Work out the finished part from the listing and answer in its coordinate system (mm). Face numbers are marked on the shaded views. A direction names the side the tool comes from. Give positions to 0.01 mm unless a question says otherwise; leave off trailing zeros. Loops run counter-clockwise (first coordinate to the right, second up) from the corner with the lowest first, then second, coordinate; pieces in that order, holes last. Notation, with made-up numbers: M 87.25,-18.5 L 101.25,-18.5 A18 ccw 101.25,-3.5 Z; hole C 0,61.5 d6. An arc over 180 degrees is marked long. Use a Markdown table: item, result.
```python
from build123d import *

# Parameters (mm, degrees)
SKETCH1_W               = 31.2625
SKETCH1_H               = 55
BOSS_EXTRUDE1_DEPTH     = 3.175
SKETCH2_R               = 1.5
CUT_EXTRUDE1_DEPTH      = 10
LPATTERN1_COUNT         = 3
LPATTERN1_PITCH         = 10
LPATTERN1_COL_COUNT     = 3
LPATTERN1_COL_PITCH     = 10
SKETCH3_W               = 6.35
SKETCH3_H               = 3.175
CUT_EXTRUDE2_DEPTH      = 10
LPATTERN2_COUNT         = 5
LPATTERN2_PITCH         = 6.35
LPATTERN2_COL_COUNT     = 5
LPATTERN2_COL_PITCH     = 6.35
SKETCH4_W               = 3.175
SKETCH4_H               = 3.6875
SKETCH4_H_2             = 3.175
CUT_EXTRUDE3_DEPTH      = 10
SKETCH5_W               = 6.35
SKETCH5_H               = 55
CUT_EXTRUDE4_DEPTH      = 10
SKETCH6_W               = 3.175
SKETCH6_H               = 3.175
CUT_EXTRUDE5_DEPTH      = 10
LPATTERN3_COUNT         = 2
LPATTERN3_PITCH         = 6.35
LPATTERN3_COUNT_DIR2    = 2
LPATTERN3_PITCH_DIR2    = 6.35
SKETCH7_W               = 5.8625
SKETCH7_H               = 3.175
CUT_EXTRUDE6_DEPTH      = 10
MIRROR1_COPY_1_SKETCH_W = 3.175
MIRROR1_COPY_1_SKETCH_H = 3.175
MIRROR1_COPY_1_DEPTH    = 10
MIRROR1_COPY_2_SKETCH_W = 3.175
MIRROR1_COPY_2_SKETCH_H = 3.175
MIRROR1_COPY_2_DEPTH    = 10
MIRROR1_COPY_3_SKETCH_W = 3.175
MIRROR1_COPY_3_SKETCH_H = 3.175
MIRROR1_COPY_3_DEPTH    = 10
SKETCH8_W               = 21.7375
SKETCH8_H               = 3.175
SKETCH8_W_2             = 3.175
SKETCH8_H_2             = 41.275
SKETCH8_W_3             = 15.875
CUT_EXTRUDE7_DEPTH      = 10
CUT_EXTRUDE8_DEPTH      = 10
LPATTERN4_COUNT         = 5
LPATTERN4_PITCH         = 10


with BuildPart() as part:
    # Sketch1 → Boss-Extrude1 (new body)
    with BuildSketch(Plane.XY):
        Rectangle(SKETCH1_W, SKETCH1_H)
    extrude(amount=BOSS_EXTRUDE1_DEPTH)

    # Sketch2 → Cut-Extrude1 (cut)
    with BuildSketch(Plane.XY.offset(3.175)):
        Circle(SKETCH2_R)
    cut_extrude1 = extrude(amount=-CUT_EXTRUDE1_DEPTH, mode=Mode.SUBTRACT)

    # LPattern1: Cut-Extrude1 ×3
    with Locations(*[(0, i * LPATTERN1_PITCH, 0) for i in range(1, LPATTERN1_COUNT)]):
        add(cut_extrude1, mode=Mode.SUBTRACT)

    # LPattern1 col: Cut-Extrude1 ×3
    with Locations(*[(0, -i * LPATTERN1_COL_PITCH, 0) for i in range(1, LPATTERN1_COL_COUNT)]):
        add(cut_extrude1, mode=Mode.SUBTRACT)

    # Sketch3 → Cut-Extrude2 (cut)
    with BuildSketch(Plane.XY.offset(3.175)):
        with Locations((15.63125, -3.175)):
            Rectangle(SKETCH3_W, SKETCH3_H)
    cut_extrude2 = extrude(amount=-CUT_EXTRUDE2_DEPTH, mode=Mode.SUBTRACT)

    # LPattern2: Cut-Extrude2 ×5
    with Locations(*[(0, i * LPATTERN2_PITCH, 0) for i in range(1, LPATTERN2_COUNT)]):
        add(cut_extrude2, mode=Mode.SUBTRACT)

    # LPattern2 col: Cut-Extrude2 ×5
    with Locations(*[(0, -i * LPATTERN2_COL_PITCH, 0) for i in range(1, LPATTERN2_COL_COUNT)]):
        add(cut_extrude2, mode=Mode.SUBTRACT)

    # Sketch4 → Cut-Extrude3 (cut)
    with BuildSketch(Plane.XY.offset(3.175)):
        with Locations((14.04375, 25.65625)):
            Rectangle(SKETCH4_W, SKETCH4_H)
        with Locations((14.04375, -25.4)):
            Rectangle(SKETCH4_W, SKETCH4_H_2)
    extrude(amount=-CUT_EXTRUDE3_DEPTH, mode=Mode.SUBTRACT)

    # Sketch5 → Cut-Extrude4 (cut)
    with BuildSketch(Plane.XY.offset(3.175)):
        with Locations((-12.45625, 0)):
            Rectangle(SKETCH5_W, SKETCH5_H)
    extrude(amount=-CUT_EXTRUDE4_DEPTH, mode=Mode.SUBTRACT)

    # Sketch6 → Cut-Extrude5 (cut)
    with BuildSketch(Plane.XY.offset(3.175)):
        with Locations((-4.51875, 25.9125)):
            Rectangle(SKETCH6_W, SKETCH6_H)
    cut_extrude5 = extrude(amount=-CUT_EXTRUDE5_DEPTH, mode=Mode.SUBTRACT)

    # LPattern3: Cut-Extrude5 2 × 2
    with Locations(*[(i * LPATTERN3_PITCH, j * LPATTERN3_PITCH_DIR2, 0) for i in range(LPATTERN3_COUNT) for j in range(LPATTERN3_COUNT_DIR2) if (i, j) != (0, 0)]):
        add(cut_extrude5, mode=Mode.SUBTRACT)

    # Sketch7 → Cut-Extrude6 (cut)
    with BuildSketch(Plane.XY.offset(3.175)):
        with Locations((9.525, 25.9125)):
            Rectangle(SKETCH7_W, SKETCH7_H)
    cut_extrude6 = extrude(amount=-CUT_EXTRUDE6_DEPTH, mode=Mode.SUBTRACT)

    # Mirror1: Cut-Extrude5, Cut-Extrude6 across plane
    add(cut_extrude5.mirror(Plane.ZX), mode=Mode.SUBTRACT)
    add(cut_extrude6.mirror(Plane.ZX), mode=Mode.SUBTRACT)

    # Mirror1 copy 1 sketch → Mirror1 copy 1 (cut)
    with BuildSketch(Plane(origin=(0, -6.35, 3.175), x_dir=(1, 0, 0), z_dir=(0, 0, 1))):
        with Locations((-4.51875, -25.9125)):
            Rectangle(MIRROR1_COPY_1_SKETCH_W, MIRROR1_COPY_1_SKETCH_H)
    extrude(amount=-MIRROR1_COPY_1_DEPTH, mode=Mode.SUBTRACT)

    # Mirror1 copy 2 sketch → Mirror1 copy 2 (cut)
    with BuildSketch(Plane(origin=(6.35, 0, 3.175), x_dir=(1, 0, 0), z_dir=(0, 0, 1))):
        with Locations((-4.51875, -25.9125)):
            Rectangle(MIRROR1_COPY_2_SKETCH_W, MIRROR1_COPY_2_SKETCH_H)
    extrude(amount=-MIRROR1_COPY_2_DEPTH, mode=Mode.SUBTRACT)

    # Mirror1 copy 3 sketch → Mirror1 copy 3 (cut)
    with BuildSketch(Plane(origin=(6.35, -6.35, 3.175), x_dir=(1, 0, 0), z_dir=(0, 0, 1))):
        with Locations((-4.51875, -25.9125)):
            Rectangle(MIRROR1_COPY_3_SKETCH_W, MIRROR1_COPY_3_SKETCH_H)
    extrude(amount=-MIRROR1_COPY_3_DEPTH, mode=Mode.SUBTRACT)

    # Sketch8 → Cut-Extrude7 (cut)
    with BuildSketch(Plane.XY.offset(3.175)):
        with Locations((1.5875, 25.9125)):
            Rectangle(SKETCH8_W, SKETCH8_H)
        with Locations((14.04375, 0)):
            Rectangle(SKETCH8_W_2, SKETCH8_H_2)
        with Locations((-1.34375, -25.9125)):
            Rectangle(SKETCH8_W_3, SKETCH8_H)
    extrude(amount=-CUT_EXTRUDE7_DEPTH, mode=Mode.SUBTRACT)

    # Sketch9 → Cut-Extrude8 (cut)
    with BuildSketch(Plane.XY.offset(3.175)):
        Polygon((3.175426481, 20), (1.58771324, 22.75), (-1.58771324, 22.75), (-3.175426481, 20), (-1.58771324, 17.25), (1.58771324, 17.25), align=None)
    cut_extrude8 = extrude(amount=-CUT_EXTRUDE8_DEPTH, mode=Mode.SUBTRACT)

    # LPattern4: Cut-Extrude8 ×5
    with Locations(*[(0, -i * LPATTERN4_PITCH, 0) for i in range(1, LPATTERN4_COUNT)]):
        add(cut_extrude8, mode=Mode.SUBTRACT)


solid = part.part
```
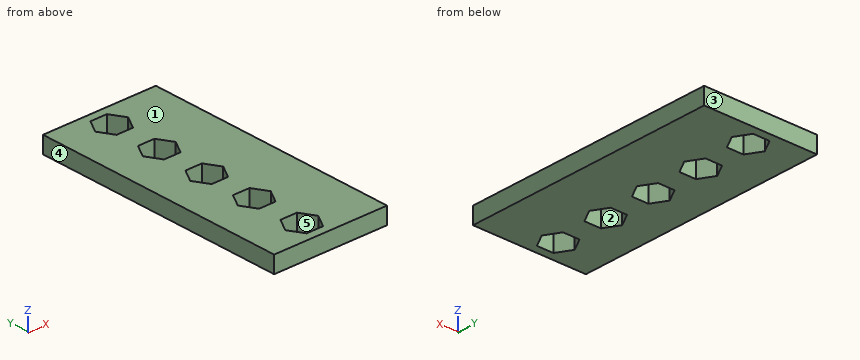
(1) A cutting plane is placed at A-A (x = 0.25). Write down the section's boundary in (y, z) (3 decimals).
Entries:
| item | result |
|---|---|
| outline | M -24.325,0 L -22.75,0 L -22.75,3.175 L -24.325,3.175 Z; M -17.25,0 L -12.75,0 L -12.75,3.175 L -17.25,3.175 Z; M -7.25,0 L -2.75,0 L -2.75,3.175 L -7.25,3.175 Z; M 2.75,0 L 7.25,0 L 7.25,3.175 L 2.75,3.175 Z; M 12.75,0 L 17.25,0 L 17.25,3.175 L 12.75,3.175 Z; M 22.75,0 L 24.325,0 L 24.325,3.175 L 22.75,3.175 Z |
(2) A cutting plane is placed at C-C (y = 18.5). Write down the section's boundary in (x, z) (3 decimals), and give its area (3 significant figures).
Entries:
| item | result |
|---|---|
| outline | M -9.281,0 L -2.309,0 L -2.309,3.175 L -9.281,3.175 Z; M 2.309,0 L 12.456,0 L 12.456,3.175 L 2.309,3.175 Z |
| area | 54.4 mm² |
(3) A cutting plane is placed at D-D (y = -2). Write down the section's boundary in (x, z) (3 decimals).
Entries:
| item | result |
|---|---|
| outline | M -9.281,0 L -2.021,0 L -2.021,3.175 L -9.281,3.175 Z; M 2.021,0 L 12.456,0 L 12.456,3.175 L 2.021,3.175 Z |
(4) The mould has two halves that part along X. Classify the marked faces 3, 4 and 5: released by +X, released by -X, zero draft, split by the parting line, or undercut.
Entries:
| item | result |
|---|---|
| face 3 | zero draft |
| face 4 | released by -X |
| face 5 | undercut |
(5) Consider probe 1 along Y at (x, z) = (1.5, 2.9) (3 decimals); probe 2 along Y at (x, z) = (2.75, 1.3) (3 decimals); probe 3 along X at (y, z) = (-12, 2.9). Determine where each line is inside the solid, lowest interval first. Write a range as [from, to].
Entries:
| item | result |
|---|---|
| probe 1 | y = [-24.325, -22.75], [-17.25, -12.75], [-7.25, -2.75], [2.75, 7.25], [12.75, 17.25], [22.75, 24.325] |
| probe 2 | y = [-24.325, -20.737], [-19.263, -10.737], [-9.263, -0.737], [0.737, 9.263], [10.737, 19.263], [20.737, 24.325] |
| probe 3 | x = [-9.28, -2.02], [2.02, 12.46] |
(6) A cutting plane is placed at B-B (z = 1.2). Count the separate pieces of the cut face and the enclosed holes in it, and give its area (3 significant figures).
Entries:
| item | result |
|---|---|
| separate pieces | 1 |
| enclosed holes | 5 |
| area | 927 mm² |
(7) Which of the six approach directions +Z, -Z, +X, -X, +Y, -Y give full straight-line access (tool end or side, diameter ignored) to the marked faces 1 and 2?
Entries:
| item | result |
|---|---|
| face 1 | +Z, +X, -X, +Y, -Y |
| face 2 | +Z, -Z |
